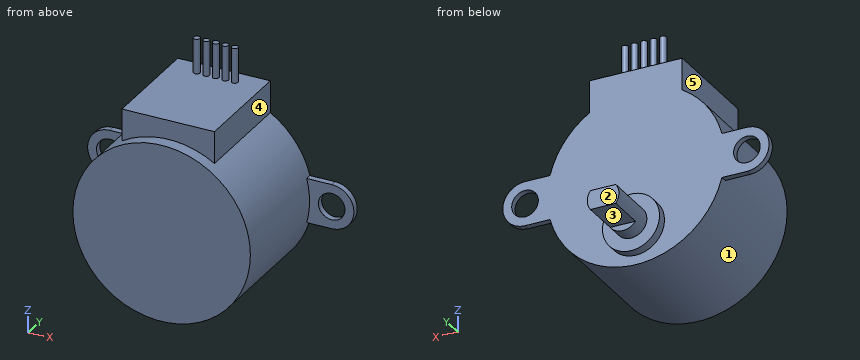
Autodesk Fusion 360 part; units mm, degrees
sketch "Skizze1" plane through (0, 0, 0) normal (0, 1, 0) x (1, 0, 0)
  circle A0 centre (0, 0) radius 14
  circle A1 centre (17.5, 0) radius 2.1
  circle A2 centre (-17.5, 0) radius 2.1
  circle A3 centre (0, 8) radius 4.5
  circle A4 centre (0, 8) radius 2.5
  line L0 (2, 9.5) -> (-2, 9.5)
  line L1 (-2, 6.5) -> (2, 6.5)
  line L2 (0, 0) -> (0, 14) construction
  line L3 (0, 0) -> (0, -17) construction
  line L4 (0, -17) -> (7.3, -17)
  line L5 (0, -17) -> (-7.3, -17)
  line L6 (-7.3, -17) -> (-7.3, -11.9461)
  line L7 (7.3, -17) -> (7.3, -11.9461)
  line L8 (0, 0) -> (-17.5, 0) construction
  line L9 (0, 0) -> (17.5, 0) construction
  line L10 (17.5, 0) -> (17.5, 3.5) construction
  line L11 (17.5, 0) -> (17.5, -3.5) construction
  line L12 (17.5, 3.5) -> (13.5554, 3.5)
  line L13 (-13.5554, 3.5) -> (-17.5, 3.5)
  arc A5 (-17.5, 3.5) -> (-17.5, -3.5) centre (-17.5, 0) ccw
  line L14 (17.5, -3.5) -> (13.5554, -3.5)
  line L15 (-13.5554, -3.5) -> (-17.5, -3.5)
  arc A6 (17.5, -3.5) -> (17.5, 3.5) centre (17.5, 0) ccw
  dimension "d1" = 28
  dimension "d2" = 4.2
  dimension "d3" = 4.2
  dimension "d4" = 17.5
  dimension "d5" = 17.5
  dimension "d6" = 9
  dimension "d7" = 8
  dimension "d8" = 5
  dimension "d9" = 3
  dimension "d10" = 17
  dimension "d11" = 7.3
  dimension "d12" = 7.3
  dimension "d13" = 7
  dimension "d14" = 7
extrude "Extrusion1" add sketch "Skizze1" against normal blind 19 contours A0 | A3 | A4 L0 L1 | A4 L0 | A4 L1
extrude "Extrusion2" add sketch "Skizze1" against normal blind 17 contours A0 L4 L5 L6 L7
extrude "Extrusion3" add sketch "Skizze1" against normal blind 1 contours A0 L12 L14 A6 | A0 L13 A5 L15
extrude "Extrusion4" add sketch "Skizze1" along normal blind 1.5 contours A3
extrude "Extrusion5" add sketch "Skizze1" along normal blind 10 contours A4 L0 L1
extrude "Extrusion6" add sketch "Skizze1" along normal blind 4 contours A4 L0 | A4 L1
sketch "Skizze2" plane through (0, 0, 17) normal (0, 0, 1) x (1, 0, 0)
  line L0 (7.3, 0) -> (-7.3, 0)
  line L1 (-7.3, 0) -> (-7.3, -17)
  line L2 (-7.3, -17) -> (7.3, -17)
  line L3 (7.3, -17) -> (7.3, 0)
  circle A0 centre (0, -2.5) radius 0.5
  circle A1 centre (-1.5, -2.5) radius 0.5
  circle A2 centre (-3, -2.5) radius 0.5
  circle A3 centre (1.5, -2.5) radius 0.5
  circle A4 centre (3, -2.5) radius 0.5
extrude "Extrusion7" add sketch "Skizze2" along normal blind 5.5 contours A0 | A1 | A2 | A3 | A4
equation "d25 = 10.00 mm - 6 mm"
Design review of the part built by this model. Coordinates are the model's own, in mm. Face numbers are marked on the shaded views. A direction names the side the tool comes from. Give positions to 0.01 mm unless a question says otherwise; leave off trailing zeros. Order: outer loops, then holes, each group sorted by start corner. A loop starts at its lowest first (then second) coordinate and runs counter-clockwise, first axis right, second up. Notation, with made-up numbers: (84.5, 31) -> (90.5, 31) arc R31 ccw to (90.5, 69) -> close; hole circle Ø4 at (52.25, 87.5). An arc over 180 degrees is marked (long way). Write item = value, one per line. Start each with the question number.
(1) We need section A-A on x = -16.5. Write out the cut boundary in (y, z).
(2) For pin 1 (3 mm diameter, centred on y = -6, z = 12, fed in from -X); pin 2 (12 mm diameter, centred on x = 15, z = -3.5, fed in from +Y); pin 3 (2 mm diameter, centred on x = 6.5, y = -1, fed in from -Z), all flat-tipped, find the tip position at first contact; note any pin that passes through.
(3) For the marked faces 1, 2, 3, 4 and 5, list the 3-axis set-ups (+Z, -Z, +X, -X, +Y, -Y) from which the entire face can be reached by the end or side of a thin tool; tool diameter is ignored.
(4) We need section B-B on y = 5.5. Write out the cut boundary in (x, z).
(5) We need section C-C on z = -8. Write out the cut boundary in (x, y), plus the area to 3 significant figures.
(6) We need section D-D on x = -8.5. Write out the cut boundary in (y, z), plus the area to 3 significant figures.
(7) To check wall thickness, follow line 1 along X through (y, z) = (-0.6, 0); line 2 along Z through (x, y) = (17.5, -0.35); line 3 along X through (y, z) = (-10.5, 14). State the ranges of each line that lie inside material, in increasing order.
Numbers:
q1.outline = (-1, -3.5) -> (0, -3.5) -> (0, -1.85) -> (-1, -1.85) -> close; (-1, 1.85) -> (0, 1.85) -> (0, 3.5) -> (-1, 3.5) -> close
q2.pin_1 = -9.26
q2.pin_2 = 0
q2.pin_3 = -12.87
q3.face_1 = -Y
q3.face_2 = +Z, -Z, +X, -X, +Y
q3.face_3 = -Z, +X, -X, +Y
q3.face_4 = +Z, +X, +Y, -Y
q3.face_5 = +Z, -X, +Y, -Y
q4.outline = (-2, -9.5) -> (2, -9.5) arc R2.5 ccw to (2, -6.5) -> (-2, -6.5) arc R2.5 ccw to start
q5.outline = (-11.49, -19) -> (11.49, -19) -> (11.49, 0) -> (4.5, 0) -> (4.5, 1.5) -> (2.5, 1.5) -> (2.5, 10) -> (-2.5, 10) -> (-2.5, 1.5) -> (-4.5, 1.5) -> (-4.5, 0) -> (-11.49, 0) -> close
q5.area = 493 mm^2
q6.outline = (-19, -11.12) -> (0, -11.12) -> (0, 11.12) -> (-19, 11.12) -> close
q6.area = 423 mm^2
q7.line_1 = -21 to -19.6, -15.4 to 15.4, 19.6 to 21
q7.line_2 = -3.5 to -2.1, 2.1 to 3.5
q7.line_3 = -7.3 to 7.3
